CAD build for the part. Positions are in the model's coordinates, mm. Round coordinates to 2 decimals unless told otherwise and drop trailing zeros. Loops run counter-clockwise (first coordinate to the right, second up) from the corner with the lowest first, then second, coordinate; pieces in that order, holes last. Notation, with made-up numbers: (65.25, 26) - (97.25, 26) arc R25 cw to (97.25, 52) - close; hole circle Ø6 at (67.5, 75). An arc over 180 degrees is marked (long way). One line per question, with ' | ' between items.
Autodesk Fusion 360 part; units mm, degrees
sketch "Sketch1" plane through (0, 0, 0) normal (0, 1, 0) x (1, 0, 0)
  line L0 (0, 0) -> (145.5, 0)
  line L1 (145.5, 0) -> (145.5, -109)
  line L2 (145.5, -109) -> (0, -109)
  line L3 (0, -109) -> (0, 0)
  line L4 (5.65, -100.6) -> (139.85, -100.6) construction
  line L5 (139.85, -100.6) -> (139.85, -8.4) construction
  line L6 (139.85, -8.4) -> (5.65, -8.4) construction
  line L7 (5.65, -8.4) -> (5.65, -100.6) construction
  circle A0 centre (5.65, -100.6) radius 2.25
  circle A1 centre (139.85, -100.6) radius 2.25
  circle A2 centre (139.85, -8.4) radius 2.25
  circle A3 centre (5.65, -8.4) radius 2.25
  line L8 (72.75, -109) -> (72.75, 0) construction
  line L9 (0, -54.5) -> (145.5, -54.5) construction
  line L10 (77.7, -15.8) -> (128, -15.8)
  line L11 (128, -15.8) -> (128, -41.1)
  line L12 (128, -41.1) -> (77.7, -41.1)
  line L13 (77.7, -41.1) -> (77.7, -15.8)
  line L14 (9.7, -26.1) -> (67.7, -26.1)
  line L15 (67.7, -26.1) -> (67.7, -18)
  line L16 (67.7, -18) -> (9.7, -18)
  line L17 (9.7, -18) -> (9.7, -26.1)
  line L18 (7.6, -74.3) -> (50.9, -74.3)
  line L19 (50.9, -74.3) -> (50.9, -63)
  line L20 (50.9, -63) -> (7.6, -63)
  line L21 (7.6, -63) -> (7.6, -74.3)
  line L22 (94.7, -74.2) -> (141.1, -74.2)
  line L23 (141.1, -74.2) -> (141.1, -63)
  line L24 (141.1, -63) -> (94.7, -63)
  line L25 (94.7, -63) -> (94.7, -74.2)
  circle A4 centre (72.75, -77.6) radius 19
  circle A5 centre (72.85, -23.45) radius 1.95
  line L26 (72.85, -25.4) -> (72.85, -21.5) construction
  line L27 (70.9, -23.45) -> (74.8, -23.45) construction
  line L28 (56.75, -93.6) -> (88.75, -93.6) construction
  line L29 (88.75, -93.6) -> (88.75, -61.6) construction
  line L30 (88.75, -61.6) -> (56.75, -61.6) construction
  line L31 (56.75, -61.6) -> (56.75, -93.6) construction
  line L32 (53.75, -77.6) -> (91.75, -77.6) construction
  circle A6 centre (56.75, -93.6) radius 1.75
  circle A7 centre (88.75, -93.6) radius 1.75
  circle A8 centre (56.75, -61.6) radius 1.75
  circle A9 centre (88.75, -61.6) radius 1.75
  line L33 (41.5, -47.8) -> (70.5, -47.8) construction
  circle A10 centre (70.5, -47.8) radius 1.9
  circle A11 centre (41.5, -47.8) radius 1.9
  line L34 (49.9, -53.4) -> (62.1, -53.4)
  line L35 (62.1, -53.4) -> (62.1, -42.2)
  line L36 (62.1, -42.2) -> (49.9, -42.2)
  line L37 (49.9, -42.2) -> (49.9, -53.4)
  line L38 (56, -53.4) -> (56, -42.2) construction
  point P0 (72.75, -96.6)
  dimension "d1" = 145.5
  dimension "d2" = 109
  dimension "d5" = 134.2
  dimension "d6" = 4.5
  dimension "d7" = 92.2
  dimension "d10" = 50.3
  dimension "d11" = 25.3
  dimension "d12" = 11.2
  dimension "d13" = 46.4
  dimension "d14" = 43.3
  dimension "d15" = 11.3
  dimension "d16" = 8.1
  dimension "d17" = 58
  dimension "d18" = 18
  dimension "d19" = 63
  dimension "d20" = 15.8
  dimension "d21" = 63
  dimension "d22" = 4.4
  dimension "d23" = 17.5
  dimension "d24" = 9.7
  dimension "d25" = 7.6
  dimension "d26" = 25.4
  dimension "d27" = 21.5
  dimension "d28" = 74.8
  dimension "d29" = 38
  dimension "d30" = 12.4
  dimension "d31" = 32
  dimension "d32" = 3.5
  dimension "d33" = 6.7
  dimension "d34" = 29
  dimension "d35" = 3.8
  dimension "d36" = 11.2
  dimension "d37" = 12.2
  dimension "d38" = 56
extrude "Extrude1" add sketch "Sketch1" along normal blind 1.8 contours L0 L1 L2 L3 | L10 L11 L12 L13 | L14 L15 L16 L17 | L18 L19 L20 L21 | L22 L23 L24 L25 | A4 | A5 | A6 | A7 | A8 | A9 | A10 | A11 | L34 L35 L36 L37 makes body 1
extrude "Extrude2" add sketch "Sketch1" along normal blind 2 separate body makes body 2
hidden bodies 1
(1) Cut at A-A, the plane z = 23.45. Write the cut outline in (x, y).
Results found:
outline: (0, 0) - (9.7, 0) - (9.7, 2) - (0, 2) - close; (67.7, 0) - (70.9, 0) - (70.9, 2) - (67.7, 2) - close; (74.8, 0) - (77.7, 0) - (77.7, 2) - (74.8, 2) - close; (128, 0) - (145.5, 0) - (145.5, 2) - (128, 2) - close
(2) Probe L1, parallel to X at y = 1.55, z = 8.4; L2, parallel to Z at x = 122, y = 0.3; L3, parallel to Z at x = 36, y = 1.2. List the from-to ranges inside material, lowest first.
Results found:
L1: x = 0 to 3.4, 7.9 to 137.6, 142.1 to 145.5 | L2: z = 0 to 15.8, 41.1 to 63, 74.2 to 109 | L3: z = 0 to 18, 26.1 to 63, 74.3 to 109
(3) Cut at B-B, the plane z = 77.6. Write the cut outline in (x, y).
Results found:
outline: (0, 0) - (53.75, 0) - (53.75, 2) - (0, 2) - close; (91.75, 0) - (145.5, 0) - (145.5, 2) - (91.75, 2) - close
(4) Cut at D-D, the plane x = 56.75. Write the cut outline in (y, z).
Results found:
outline: (0, 0) - (2, 0) - (2, 18) - (0, 18) - close; (0, 26.1) - (2, 26.1) - (2, 42.2) - (0, 42.2) - close; (0, 53.4) - (2, 53.4) - (2, 59.85) - (0, 59.85) - close; (0, 63.35) - (2, 63.35) - (2, 67.35) - (0, 67.35) - close; (0, 87.85) - (2, 87.85) - (2, 91.85) - (0, 91.85) - close; (0, 95.35) - (2, 95.35) - (2, 109) - (0, 109) - close
(5) Drop a flat-ended pin along its axis: P1, Ø3, axis at x = 88.75, z = 93.6, coming from the +Y side. Give the stop position or say it passes through.
Results found:
P1: passes through
(6) Cut at C-C, the plane x = 126. Write the cut outline in (y, z).
Results found:
outline: (0, 0) - (2, 0) - (2, 15.8) - (0, 15.8) - close; (0, 41.1) - (2, 41.1) - (2, 63) - (0, 63) - close; (0, 74.2) - (2, 74.2) - (2, 109) - (0, 109) - close
(7) Two-plate mould, pull along Z, no slides. Class faces 1 (the face through (70.253, 0.986, 49.684)), 2 (the face through (72, 0, 54)): released by +Z, released by -Z, zero draft, split by the parting line, or undercut.
Results found:
face 1: undercut | face 2: zero draft
